Model file for the job. Use its own axes, mm. Coordinates: 2 decimals unless noted, no trailing zeros. Order: outer loops, then holes, each group sorted by start corner. A loop starts at its lowest first (then second) coordinate and runs counter-clockwise, first axis right, second up. Notation, with made-up numbers: (53, 76.25) -> (72, 76.25) arc R11 ccw to (72, 85.25) -> close; hole circle Ø8 at (-20.75, 5). An arc over 180 degrees is marked (long way). Use CSV: the item, a comma, the result in double quotes. Start each with the question number.
(1) Cut at B-B on z = -13. Give the number of separate pieces and of enclosed holes in the cut face, plus the area to 3 significant figures.
(2) Cut at A-A on x = 0. Write the cut outline in (y, z), plus the area to 3 significant figures.
(3) Pull direction X, two halves, no side cores. Call faces 1 (the flat face through (7.5, 0, -17)), 2 (the flat face through (2, 23, -0.75)), 3 (the cylindrical face through (0.32, -17.562, -9.165)): pulls with the +X half, pulls with the -X half, needs draft (parallel to the pull), parting line crosses it, or undercut.
(4) Probe L1, parallel to X at y = 20, z = -10.25; L2, parallel to Y at x = 2, z = -17; L3, parallel to Y at x = 0, z = -7.25. List the from-to ranges inside material, lowest first.
(5) Cut at C-C on x = 4.5. Write the cut outline in (y, z), plus the area to 3 significant figures.
(6) Pin check, flat tips, straight feed: pin 1 Ø4 at (x, y) = (0, 20) entering from +Z; pin 2 Ø8 at (x, y) = (2.5, 4.5) entering from +Z; pin 3 Ø4 at (x, y) = (1.5, 8) entering from +Z; pin 4 Ø1.5 at (x, y) = (-3, 6) entering from +Z. Stop position of each tip, or through.
```python
from build123d import *

# Parameters (mm, degrees)
BOSS_EXTRUDE1_DEPTH = 15
CUT_EXTRUDE1_DEPTH  = 42.676582154
HOLE1_D             = 4.917
HOLE1_DEPTH         = 26.75
CHAMFER1_SIZE       = 0.5415


with BuildPart() as part:
    # Sketch1 → Boss-Extrude1 (new body)
    with BuildSketch(Plane(origin=(7.5, 0, 0), x_dir=(0, 0, -1), z_dir=(1, 0, 0))):
        with BuildLine():
            Line((0.75, 27.489770825), (0.75, -27.489770825))
            ThreePointArc((0.75, -27.489770825), (27.5, 0), (0.75, 27.489770825))
        make_face()
    extrude(amount=-BOSS_EXTRUDE1_DEPTH)

    # Sketch2 → Cut-Extrude1 (cut, through all)
    with BuildSketch(Plane.ZY.offset(7.5)):
        with BuildLine():
            Line((-0.75, -14.981238267), (-0.75, 14.981238267))
            ThreePointArc((-0.75, 14.981238267), (-15, 0), (-0.75, -14.981238267))
        make_face()
    extrude(amount=-CUT_EXTRUDE1_DEPTH, mode=Mode.SUBTRACT)

    # Hole1
    with Locations(Plane.XY.offset(-0.75)):
        with Locations((0, -20), (0, 20)):
            Hole(HOLE1_D / 2, depth=HOLE1_DEPTH)

    # Chamfer1
    chamfer1_edges = [part.edges().sort_by_distance(p)[0] for p in [
        (7.5, 0, -15),
        (-7.5, 0, -15),
        (2.4585, 20, -0.75),
        (2.4585, -20, -0.75),
        (7.5, 0, -27.5),
        (-7.5, 0, -27.5),
    ]]
    chamfer(chamfer1_edges, length=CHAMFER1_SIZE)


solid = part.part
```
Outcome:
1,separate pieces,"2"
1,enclosed holes,"2"
1,area,"463 mm2"
2,outline,"(-27.49, -0.75) arc R27.5 ccw to (-22.46, -15.87) -> (-22.46, -1.29) -> (-23, -0.75) -> close; (-17.54, -21.18) arc R27.5 ccw to (17.54, -21.18) -> (17.54, -1.29) -> (17, -0.75) -> (14.98, -0.75) arc R15 cw to (-14.98, -0.75) -> (-17, -0.75) -> (-17.54, -1.29) -> close; (22.46, -15.87) arc R27.5 ccw to (27.49, -0.75) -> (23, -0.75) -> (22.46, -1.29) -> close"
2,area,"638 mm2"
3,face 1,"pulls with the +X half"
3,face 2,"needs draft"
3,face 3,"undercut"
4,L1,"-7.5 to -2.46, 2.46 to 7.5"
4,L2,"-21.62 to -21.43, -18.57 to 18.57, 21.43 to 21.62"
4,L3,"-26.53 to -22.46, -17.54 to -13.13, 13.13 to 17.54, 22.46 to 26.53"
5,outline,"(-27.49, -0.75) arc R27.5 ccw to (27.49, -0.75) -> (14.98, -0.75) arc R15 cw to (-14.98, -0.75) -> close"
5,area,"816 mm2"
6,pin 1,"through"
6,pin 2,"z = -12.36"
6,pin 3,"z = -11.18"
6,pin 4,"z = -13.4"
